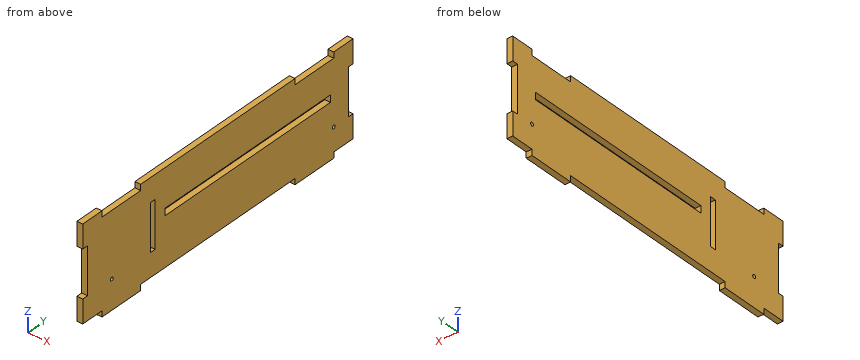
```python
from build123d import *

# Parameters (mm, degrees)
F0_W      = 355.6
F0_H      = 101.6
F1_DEPTH  = 6.35
F2_W      = 50.8
F2_H      = 6.35
F3_DEPTH  = 6.35
F4_R      = 1.905
F5_DEPTH  = 6.351
F6_W      = 6.35
F6_H      = 50.8
F7_DEPTH  = 25.4
F9_W      = 6.35
F9_H      = 50.8
F10_DEPTH = 25.4
F11_W     = 50.8
F11_H     = 6.35
F12_DEPTH = 25.4
F13_W     = 217.805
F13_H     = 7.62
F14_DEPTH = 25.4


with BuildPart() as f1:
    # F0 (on Right) → F1 (new body)
    with BuildSketch(Plane.YZ):
        with Locations((0, 50.8)):
            Rectangle(F0_W, F0_H)
    extrude(amount=F1_DEPTH)

    # F4 (on face) → F5 (cut, through all)
    with BuildSketch(Plane.YZ.offset(6.35)):
        with Locations((152.4, 25.4)):
            Circle(F4_R)
        with Locations((-139.7, 25.4)):
            Circle(F4_R)
    extrude(amount=-F5_DEPTH, mode=Mode.SUBTRACT)

    # F6 (on face) → F7 (cut)
    with BuildSketch(Plane.YZ.offset(6.35)):
        with Locations((174.625, 50.8)):
            Rectangle(F6_W, F6_H)
        with Locations((-174.625, 50.8)):
            Rectangle(F6_W, F6_H)
    extrude(amount=-F7_DEPTH, mode=Mode.SUBTRACT)


with BuildPart() as f3:
    # F2 (on face) → F3 (new body)
    with BuildSketch(Plane.YZ.offset(6.35)):
        with Locations((127, -3.175)):
            Rectangle(F2_W, F2_H)
        with Locations((-127, -3.175)):
            Rectangle(F2_W, F2_H)
    extrude(amount=-F3_DEPTH)

    # F8: union F1
    add(f1.part)

    # F9 (on face) → F10 (cut)
    with BuildSketch(Plane.YZ.offset(6.35)):
        with Locations((-85.725, 50.8)):
            Rectangle(F9_W, F9_H)
    extrude(amount=-F10_DEPTH, mode=Mode.SUBTRACT)

    # F11 (on face) → F12 (cut)
    with BuildSketch(Plane.YZ.offset(6.35)):
        with Locations((-127, 98.425)):
            Rectangle(F11_W, F11_H)
        with Locations((127, 98.425)):
            Rectangle(F11_W, F11_H)
    extrude(amount=-F12_DEPTH, mode=Mode.SUBTRACT)

    # F13 (on face) → F14 (cut)
    with BuildSketch(Plane.YZ.offset(6.35)):
        with Locations((39.0525, 56.515)):
            Rectangle(F13_W, F13_H)
    extrude(amount=-F14_DEPTH, mode=Mode.SUBTRACT)


solid = f3.part
```
CAD build for the part. Positions are in the model's coordinates, mm. Round coordinates to 2 decimals unless told otherwise and drop trailing zeros. Write each loop counter-clockwise with the first axis right and the second up, starting at its lowest first coordinate (ties: lowest second). Pieces come first, ordered by that corner, then holes. Notation, with made-up numbers: (62, 16) -> (105, 16) arc R13 cw to (105, 25) -> close; hole circle Ø10 at (-28, -37). An arc over 180 degrees is marked (long way). Answer in a Markdown table with one row per item. Add a question column.
Item 1: Saw through at C-C, the plane x = 1.5. Count the separate pieces of the cut face and the enclosed holes in it, then the cut area to 3 significant figures.
Item 2: Drill centre lines: line 1 (Z direction, x = 0.75, y = 9.5) (3 decimals); line 2 (Z direction, x = 3.25, y = -139.7) (3 decimals); line 3 (Y direction, x = 3.25, z = 41.5). Where is each one in solid material? Low to high. Write a range as from..to.
Item 3: Saw through at D-D, the plane y = -75. Write the cut outline in (x, z).
Item 4: Drop flat-ended pins along their axis: pin 1 Ø1.9 at (x, z) = (4.5, -3.5) entering from -Y; pin 2 Ø1.9 at (x, z) = (3.5, 42.5) entering from +Y; pin 3 Ø3 at (y, z) = (-133.5, 53.5) entering from -X; pin 4 Ø3 at (x, z) = (1.5, -2) entering from +Y. Give the stop position or say it passes through.
Item 5: Saw through at B-B, the plane z = 63.5. Write the cut outline in (x, y).
Item 6: Saw through at A-A, the plane y = 127. Write the cut outline in (x, z) (3 decimals).
Findings below:
| question | item | result |
|---|---|---|
| 1 | separate pieces | 1 |
| 1 | enclosed holes | 4 |
| 1 | area | 33,500 mm^2 |
| 2 | line 1 | z = 0..52.705, 60.325..101.6 |
| 2 | line 2 | z = -6.35..23.495, 27.305..95.25 |
| 2 | line 3 | y = -171.45..-88.9, -82.55..171.45 |
| 3 | outline | (0, 0) -> (6.35, 0) -> (6.35, 101.6) -> (0, 101.6) -> close |
| 4 | pin 1 | stops at y = -152.4 |
| 4 | pin 2 | stops at y = 171.45 |
| 4 | pin 3 | stops at x = 0 |
| 4 | pin 4 | stops at y = 152.4 |
| 5 | outline | (0, -171.45) -> (6.35, -171.45) -> (6.35, -88.9) -> (0, -88.9) -> close; (0, -82.55) -> (6.35, -82.55) -> (6.35, 171.45) -> (0, 171.45) -> close |
| 6 | outline | (0, -6.35) -> (6.35, -6.35) -> (6.35, 52.705) -> (0, 52.705) -> close; (0, 60.325) -> (6.35, 60.325) -> (6.35, 95.25) -> (0, 95.25) -> close |
